Read the model definition and answer for the solid it produces. Units are mm, in the model's axes. A direction names the side the tool comes from. Give positions to 0.01 mm unless a question says otherwise; leave off trailing zeros. Order: outer loops, then holes, each group sorted by start corner. A loop starts at its lowest first (then second) coordinate and runs counter-clockwise, first axis right, second up. Notation, with made-up numbers: M 70,80.25 L 106,80.25 A14 cw 106,95.25 Z; hole C 33,-14 d6. An arc over 180 degrees is marked long. Write item = value, one per line. Start each with the question number.
Autodesk Inventor part; units mm, degrees
ref_plane "YZ Plane" through (0, 0, 0) normal (1, 0, 0) x (0, 1, 0)
ref_plane "XZ Plane" through (0, 0, 0) normal (0, 1, 0) x (-1, 0, 0)
ref_plane "XY Plane" through (0, 0, 0) normal (0, 0, 1) x (1, 0, 0)
sketch "草圖1" plane through (0, 0, 0) normal (0, 1, 0) x (-1, 0, 0)
  line L0 (-8, 28) -> (-8, -28)
  line L1 (-8, -28) -> (8, -28)
  line L2 (8, -28) -> (8, 28)
  line L3 (8, 28) -> (-8, 28)
  line L4 (-8, 28) -> (8, -28) construction
  line L5 (-8, -28) -> (8, 28) construction
  line L6 (-7, 27) -> (-7, -27)
  line L7 (-7, -27) -> (7, -27)
  line L8 (7, -27) -> (7, 27)
  line L9 (7, 27) -> (-7, 27)
  line L10 (-7, 27) -> (7, -27) construction
  line L11 (-7, -27) -> (7, 27) construction
  line L12 (7, 27) -> (8, 27)
  line L13 (7, -27) -> (8, -27)
  point P0 (0, 0)
  dimension "d0" = 56
  dimension "d1" = 16
  dimension "d2" = 54
  dimension "d3" = 14
extrude "擠出1" add sketch "草圖1" along normal blind 2 contours L3 L2 L12 L9 L6 L7 L13 L1 L0
fillet "圓角1" radius 0.2 6 edges at (0, 2, 27) (7, 2, 0) (8, 2, 0) (0, 2, 28) (0, 2, -27) (0, 2, -28)
properties part number "矮牆"
1) Find section C-C on z = -21. Determine the outline of the cut face in (x, y), plus the area to 3 significant figures.
2) Find section B-B on y = 0.9. Determine the outline of the cut face in (x, z), plus the area to 3 significant figures.
3) For a pull along Z with two mould halves and no side action, classify faces 1 (the face through (7, 1, 0)), 2 (the face through (8, 1, 0)), 3 (the face through (0, 1, -28)) as pulls with the +Z half, pulls with the -Z half, needs draft (parallel to the pull), parting line crosses it, or undercut.
4) Find the intervals of material crossed by probe 1 along Z at (x, y) = (-0.5, 1.8); probe 2 along X at (y, z) = (0.45, 9), in increasing order. Write a range as [from, to].
5) This flat-tipped pin is pushed along its axis until it touches: P1, Ø0.5, axis at y = 0.5, z = 7.5, coming from the -X side. Where does it stop, or does it pass through?
6) For faces 4 (the face through (-8, 1, -27.5)), 5 (the face through (0, 1, -27)), determine the directions among +Z, -Z, +X, -X, +Y, -Y from which every point of the face is accessible in a straight line to the end or side of a thin tool.
7) Find section A-A on x = 3.5. Determine the outline of the cut face in (y, z), plus the area to 3 significant figures.
Numbers:
q1.outline = M 7,0 L 8,0 L 8,1.8 A0.2 ccw 7.8,2 L 7.2,2 A0.2 ccw 7,1.8 Z
q1.area = 1.98 mm2
q2.outline = M -8,-28 L 8,-28 L 8,28 L -8,28 L -8,27 L 7,27 L 7,-27 L -8,-27 Z
q2.area = 86.0 mm2
q3.face_1 = undercut
q3.face_2 = needs draft
q3.face_3 = pulls with the -Z half
q4.probe_1 = [-28, -27], [27, 28]
q4.probe_2 = [7, 8]
q5.P1 = 7
q6.face_4 = +Z, -Z, -X, +Y, -Y
q6.face_5 = -X, +Y, -Y
q7.outline = M 0,-28 L 1.8,-28 A0.2 ccw 2,-27.8 L 2,-27.2 A0.2 ccw 1.8,-27 L 0,-27 Z; M 0,27 L 1.8,27 A0.2 ccw 2,27.2 L 2,27.8 A0.2 ccw 1.8,28 L 0,28 Z
q7.area = 3.97 mm2
